from build123d import *

# Parameters (mm, degrees)
BASPROSKE_W         = 6
BASPROSKE_H         = 20.25
TOOTHCUT_DEPTH      = 30.259613805
TEETHCUTS_COUNT     = 25
TEETHCUTS_ANGLE     = 345.6
BORSKE_R            = 0.4
BORE_DEPTH          = 50.0000508
SKETCH1_R           = 0.4
BOSS_EXTRUDE1_DEPTH = 6


with BuildPart() as part:
    # BasProSke → Base-Revolve (revolve)
    with BuildSketch(Plane(origin=(0, 0, 0), x_dir=(1, 0, 0), z_dir=(0, 1, 0)), mode=Mode.PRIVATE) as base_revolve_sk:
        with Locations((3, 10.125)):
            Rectangle(BASPROSKE_W, BASPROSKE_H)
    revolve(base_revolve_sk.sketch.rotate(Axis((-10, 0, 0), (1, 0, 0)), 180), axis=Axis((-10, 0, 0), (1, 0, 0)))

    # TooCutSke → ToothCut (cut, through all)
    with BuildSketch(Plane(origin=(0, 0, 0), x_dir=(0, 0, -1), z_dir=(1, 0, 0))):
        with BuildLine():
            ThreePointArc((0.713909619, 16.858891098), (0, 16.874), (-0.713909619, 16.858891098))
            ThreePointArc((-0.713909619, 16.858891098), (-1.221902209, 18.597177626), (-2.131751691, 20.163022588))
            ThreePointArc((-2.131751691, 20.163022588), (0, 20.2754), (2.131751691, 20.163022588))
            ThreePointArc((2.131751691, 20.163022588), (1.221902209, 18.597177626), (0.713909619, 16.858891098))
        make_face()
    toothcut = extrude(amount=TOOTHCUT_DEPTH, mode=Mode.SUBTRACT)

    # TeethCuts: ToothCut ×25 about axis
    teethcuts_axis = Axis((-10, 0, 0), (1, 0, 0))
    for i in range(1, TEETHCUTS_COUNT):
        add(toothcut.rotate(teethcuts_axis, i * TEETHCUTS_ANGLE / (TEETHCUTS_COUNT - 1)), mode=Mode.SUBTRACT)

    # BorSke → Bore (cut, symmetric)
    with BuildSketch(Plane(origin=(0, 0, 0), x_dir=(0, 0, -1), z_dir=(1, 0, 0))):
        with Locations(Location((0, 0, 0), (0, 0, 180))):
            Circle(BORSKE_R)
    extrude(amount=BORE_DEPTH, both=True, mode=Mode.SUBTRACT)

    # Sketch1 → Boss-Extrude1 (add)
    with BuildSketch(Plane(origin=(6, 0, 0), x_dir=(0, 0, -1), z_dir=(1, 0, 0))):
        with BuildLine():
            ThreePointArc((7.033321313, 19.122578704), (5.755923301, 17.845039552), (4.814939591, 16.302832813))
            ThreePointArc((4.814939591, 16.302832813), (4.227479392, 16.464945156), (3.634585878, 16.605896136))
            ThreePointArc((3.634585878, 16.605896136), (3.55295933, 18.410664563), (3.049026099, 20.145571842))
            ThreePointArc((3.049026099, 20.145571842), (2.553664634, 20.214337039), (2.056764651, 20.270923614))
            ThreePointArc((2.056764651, 20.270923614), (1.137209513, 18.715844736), (0.609319757, 16.988076125))
            ThreePointArc((0.609319757, 16.988076125), (0, 16.999), (-0.609319757, 16.988076125))
            ThreePointArc((-0.609319757, 16.988076125), (-1.137209513, 18.715844736), (-2.056764651, 20.270923614))
            ThreePointArc((-2.056764651, 20.270923614), (-2.553664634, 20.214337039), (-3.049026099, 20.145571842))
            ThreePointArc((-3.049026099, 20.145571842), (-3.55295933, 18.410664563), (-3.634585878, 16.605896136))
            ThreePointArc((-3.634585878, 16.605896136), (-4.227479392, 16.464945156), (-4.814939591, 16.302832813))
            ThreePointArc((-4.814939591, 16.302832813), (-5.755923301, 17.845039552), (-7.033321313, 19.122578704))
            ThreePointArc((-7.033321313, 19.122578704), (-7.500537761, 18.9441959), (-7.963235326, 18.754399701))
            ThreePointArc((-7.963235326, 18.754399701), (-8.019882673, 16.948674626), (-7.650117116, 15.180306621))
            ThreePointArc((-7.650117116, 15.180306621), (-8.189330706, 14.896337254), (-8.718019063, 14.593222558))
            ThreePointArc((-8.718019063, 14.593222558), (-10.012971259, 15.852964904), (-11.567948531, 16.772691847))
            ThreePointArc((-11.567948531, 16.772691847), (-11.976124515, 16.48372126), (-12.37708519, 16.184819653))
            ThreePointArc((-12.37708519, 16.184819653), (-11.982887291, 14.421737129), (-11.18496336, 12.800882612))
            ThreePointArc((-11.18496336, 12.800882612), (-11.636616254, 12.391737698), (-12.073313334, 11.966666459))
            ThreePointArc((-12.073313334, 11.966666459), (-13.640867407, 12.864790167), (-15.375718999, 13.368915074))
            ThreePointArc((-15.375718999, 13.368915074), (-15.699207322, 12.987513791), (-16.013237272, 12.598287862))
            ThreePointArc((-16.013237272, 12.598287862), (-15.192963031, 10.988628849), (-14.01701722, 9.61713207))
            ThreePointArc((-14.01701722, 9.61713207), (-14.352730406, 9.108519688), (-14.669996926, 8.588200696))
            ThreePointArc((-14.669996926, 8.588200696), (-16.411657689, 9.068273351), (-18.217376494, 9.125120201))
            ThreePointArc((-18.217376494, 9.125120201), (-18.435851194, 8.675253066), (-18.643218764, 8.220159312))
            ThreePointArc((-18.643218764, 8.220159312), (-17.448409029, 6.865064605), (-15.968330338, 5.82910175))
            ThreePointArc((-15.968330338, 5.82910175), (-16.167009721, 5.252979887), (-16.344910658, 4.670106699))
            ThreePointArc((-16.344910658, 4.670106699), (-18.15124316, 4.70196357), (-19.914369225, 4.307960465))
            ThreePointArc((-19.914369225, 4.307960465), (-20.014102734, 3.817894285), (-20.101778256, 3.32552792))
            ThreePointArc((-20.101778256, 3.32552792), (-18.607507316, 2.310143104), (-16.916294533, 1.674807529))
            ThreePointArc((-16.916294533, 1.674807529), (-16.965456357, 1.067376041), (-16.992813542, 0.458572722))
            ThreePointArc((-16.992813542, 0.458572722), (-18.750319268, 0.040212124), (-20.360068898, -0.77988427))
            ThreePointArc((-20.360068898, -0.77988427), (-20.334794592, -1.279356835), (-20.297269091, -1.778058621))
            ThreePointArc((-20.297269091, -1.778058621), (-18.597427484, -2.389933184), (-16.801345729, -2.584721008))
            ThreePointArc((-16.801345729, -2.584721008), (-16.697900975, -3.185294967), (-16.572995455, -3.781775066))
            ThreePointArc((-16.572995455, -3.781775066), (-18.171243857, -4.624065996), (-19.526470563, -5.818726009))
            ThreePointArc((-19.526470563, -5.818726009), (-19.37777652, -6.29622126), (-19.21740786, -6.769923199))
            ThreePointArc((-19.21740786, -6.769923199), (-17.418802888, -6.939841181), (-15.630706582, -6.681842018))
            ThreePointArc((-15.630706582, -6.681842018), (-15.381155065, -7.237822177), (-15.111835113, -7.784500017))
            ThreePointArc((-15.111835113, -7.784500017), (-16.450402366, -8.997797045), (-17.465952269, -10.491955792))
            ThreePointArc((-17.465952269, -10.491955792), (-17.203181482, -10.917470948), (-16.930046218, -11.336408605))
            ThreePointArc((-16.930046218, -11.336408605), (-15.145690844, -11.053693433), (-13.477932654, -10.35911832))
            ThreePointArc((-13.477932654, -10.35911832), (-13.097954614, -10.835570402), (-12.701142593, -11.298096204))
            ThreePointArc((-12.701142593, -11.298096204), (-13.695921594, -12.806163413), (-14.307983958, -14.505937407))
            ThreePointArc((-14.307983958, -14.505937407), (-13.947647283, -14.852735784), (-13.578907507, -15.190585766))
            ThreePointArc((-13.578907507, -15.190585766), (-11.920919342, -14.473001475), (-10.47829065, -13.38549312))
            ThreePointArc((-10.47829065, -13.38549312), (-9.991761504, -13.752479887), (-9.492390573, -14.101791454))
            ThreePointArc((-9.492390573, -14.101791454), (-10.080875698, -15.809871436), (-10.250992395, -17.608457625))
            ThreePointArc((-10.250992395, -17.608457625), (-9.81573111, -17.854748606), (-9.374556097, -18.090282557))
            ThreePointArc((-9.374556097, -18.090282557), (-7.947112637, -16.982917606), (-6.820259107, -15.570808159))
            ThreePointArc((-6.820259107, -15.570808159), (-6.257749271, -15.805270484), (-5.687196742, -16.019419285))
            ThreePointArc((-5.687196742, -16.019419285), (-5.832411307, -17.820187093), (-5.549893279, -19.604573691))
            ThreePointArc((-5.549893279, -19.604573691), (-5.067056451, -19.734881908), (-4.581166851, -19.853300363))
            ThreePointArc((-4.581166851, -19.853300363), (-3.473959616, -18.425734565), (-2.733685602, -16.777752055))
            ThreePointArc((-2.733685602, -16.777752055), (-2.130539637, -16.864957808), (-1.524655424, -16.930488086))
            ThreePointArc((-1.524655424, -16.930488086), (-1.217475063, -18.710794856), (-0.500073957, -20.368862291))
            ThreePointArc((-0.500073957, -20.368862291), (0, -20.375), (0.500073957, -20.368862291))
            ThreePointArc((0.500073957, -20.368862291), (1.217475063, -18.710794856), (1.524655424, -16.930488086))
            ThreePointArc((1.524655424, -16.930488086), (2.130539637, -16.864957808), (2.733685602, -16.777752055))
            ThreePointArc((2.733685602, -16.777752055), (3.473959616, -18.425734565), (4.581166851, -19.853300363))
            ThreePointArc((4.581166851, -19.853300363), (5.067056451, -19.734881908), (5.549893279, -19.604573691))
            ThreePointArc((5.549893279, -19.604573691), (5.832411307, -17.820187093), (5.687196742, -16.019419285))
            ThreePointArc((5.687196742, -16.019419285), (6.257749271, -15.805270484), (6.820259107, -15.570808159))
            ThreePointArc((6.820259107, -15.570808159), (7.947112637, -16.982917606), (9.374556097, -18.090282557))
            ThreePointArc((9.374556097, -18.090282557), (9.81573111, -17.854748606), (10.250992395, -17.608457625))
            ThreePointArc((10.250992395, -17.608457625), (10.080875698, -15.809871436), (9.492390573, -14.101791454))
            ThreePointArc((9.492390573, -14.101791454), (9.991761504, -13.752479887), (10.47829065, -13.38549312))
            ThreePointArc((10.47829065, -13.38549312), (11.920919342, -14.473001475), (13.578907507, -15.190585766))
            ThreePointArc((13.578907507, -15.190585766), (13.947647283, -14.852735784), (14.307983958, -14.505937407))
            ThreePointArc((14.307983958, -14.505937407), (13.695921594, -12.806163413), (12.701142593, -11.298096204))
            ThreePointArc((12.701142593, -11.298096204), (13.097954614, -10.835570402), (13.477932654, -10.35911832))
            ThreePointArc((13.477932654, -10.35911832), (15.145690844, -11.053693433), (16.930046218, -11.336408605))
            ThreePointArc((16.930046218, -11.336408605), (17.203181482, -10.917470948), (17.465952269, -10.491955792))
            ThreePointArc((17.465952269, -10.491955792), (16.450402366, -8.997797045), (15.111835113, -7.784500017))
            ThreePointArc((15.111835113, -7.784500017), (15.381155065, -7.237822177), (15.630706582, -6.681842018))
            ThreePointArc((15.630706582, -6.681842018), (17.418802888, -6.939841181), (19.21740786, -6.769923199))
            ThreePointArc((19.21740786, -6.769923199), (19.37777652, -6.29622126), (19.526470563, -5.818726009))
            ThreePointArc((19.526470563, -5.818726009), (18.171243857, -4.624065996), (16.572995455, -3.781775066))
            ThreePointArc((16.572995455, -3.781775066), (16.697900975, -3.185294967), (16.801345729, -2.584721008))
            ThreePointArc((16.801345729, -2.584721008), (18.597427484, -2.389933184), (20.297269091, -1.778058621))
            ThreePointArc((20.297269091, -1.778058621), (20.334794592, -1.279356835), (20.360068898, -0.77988427))
            ThreePointArc((20.360068898, -0.77988427), (18.750319268, 0.040212124), (16.992813542, 0.458572722))
            ThreePointArc((16.992813542, 0.458572722), (16.965456357, 1.067376041), (16.916294533, 1.674807529))
            ThreePointArc((16.916294533, 1.674807529), (18.607507316, 2.310143104), (20.101778256, 3.32552792))
            ThreePointArc((20.101778256, 3.32552792), (20.014102734, 3.817894285), (19.914369225, 4.307960465))
            ThreePointArc((19.914369225, 4.307960465), (18.15124316, 4.70196357), (16.344910658, 4.670106699))
            ThreePointArc((16.344910658, 4.670106699), (16.167009721, 5.252979887), (15.968330338, 5.82910175))
            ThreePointArc((15.968330338, 5.82910175), (17.448409029, 6.865064605), (18.643218764, 8.220159312))
            ThreePointArc((18.643218764, 8.220159312), (18.435851194, 8.675253066), (18.217376494, 9.125120201))
            ThreePointArc((18.217376494, 9.125120201), (16.411657689, 9.068273351), (14.669996926, 8.588200696))
            ThreePointArc((14.669996926, 8.588200696), (14.352730406, 9.108519688), (14.01701722, 9.61713207))
            ThreePointArc((14.01701722, 9.61713207), (15.192963031, 10.988628849), (16.013237272, 12.598287862))
            ThreePointArc((16.013237272, 12.598287862), (15.699207322, 12.987513791), (15.375718999, 13.368915074))
            ThreePointArc((15.375718999, 13.368915074), (13.640867407, 12.864790167), (12.073313334, 11.966666459))
            ThreePointArc((12.073313334, 11.966666459), (11.636616254, 12.391737698), (11.18496336, 12.800882612))
            ThreePointArc((11.18496336, 12.800882612), (11.982887291, 14.421737129), (12.37708519, 16.184819653))
            ThreePointArc((12.37708519, 16.184819653), (11.976124515, 16.48372126), (11.567948531, 16.772691847))
            ThreePointArc((11.567948531, 16.772691847), (10.012971259, 15.852964904), (8.718019063, 14.593222558))
            ThreePointArc((8.718019063, 14.593222558), (8.189330706, 14.896337254), (7.650117116, 15.180306621))
            ThreePointArc((7.650117116, 15.180306621), (8.019882673, 16.948674626), (7.963235326, 18.754399701))
            ThreePointArc((7.963235326, 18.754399701), (7.500537761, 18.9441959), (7.033321313, 19.122578704))
        make_face()
        with Locations(Location((0, 0, 0), (0, 0, 180))):
            Circle(SKETCH1_R, mode=Mode.SUBTRACT)
    extrude(amount=-BOSS_EXTRUDE1_DEPTH)


solid = part.part
CAD build for the part. Positions are in the model's coordinates, mm. A direction names the side the tool comes from. Give positions to 0.01 mm unless a question says otherwise; leave off trailing zeros. Loops run counter-clockwise (first coordinate to the right, second up) from the corner with the lowest first, then second, coordinate; pieces in that order, holes last. Notation, with made-up numbers: M 28.5,27 L 60.5,27 A6 cw 60.5,31 Z; hole C 75,82 d7. An arc over 180 degrees is marked long. Write each question's results on one line, items separated by ' | '.
Q1. Mould opens along Z. For faces 1 (the face through (6, -4, 0)), 2 (the face through (3.042, 3.811, -20.015)), 3 (the face through (3.04, 12.4, 11.63)) say: pulls with the +Z half, pulls with the -Z half, needs draft (parallel to the pull), parting line crosses it, or undercut.
Geometry check:
face 1: needs draft | face 2: pulls with the -Z half | face 3: undercut
Q2. Band-saw the part on A-A on y = 11.5. Write the cut outline in (x, z).
Geometry check:
outline: M 0,-15.51 L 6,-15.51 L 6,15.51 L 0,15.51 Z
Q3. Band-saw the part on B-B on y = 6.5. Write the cut outline in (x, z).
Geometry check:
outline: M 0,-17.01 L 6,-17.01 L 6,17.01 L 0,17.01 Z
Q4. Probe probe 1 along Y at (x, z) = (2.6, 0) (3 decimals); probe 2 along Y at (x, z) = (3.6, 17.5); probe 3 along Z at (x, y) = (2.2, 16). List the from-to ranges inside material, lowest first.
Geometry check:
probe 1: y = -20.375 to -0.4, 0.4 to 16.999 | probe 2: y = -6.94 to -4.21, -2.56 to 0.38, 1.84 to 4.74, 6.91 to 9.15 | probe 3: z = -12.36 to -10.21, -7.88 to 7.88, 10.21 to 12.36
Q5. Which spindle directions (+Z, -Z, +X, -X, +Y, -Y) get a long thin tool onto all of the face, cutting with end or side? Do faces 4 (the face through (3, 11, -15.2)), 5 (the face through (3.042, 14.446, 11.991)), 6 (the face through (3.042, 17.825, 5.74)). Say none if no direction does.
Geometry check:
face 4: -Z, +X, -X | face 5: +X, -X | face 6: +X, -X, +Y
Q6. Flat gauge pins, fed straight in: P1, Ø1, axis at x = 2, z = -7.5, coming from the -Y side; P2, Ø3, axis at y = 13.5, z = -5, coming from the -X side; P3, Ø1.5, axis at x = 5.5, z = 11.5, coming from the +Y side. Where does each tip first touch, or does it go through?
Geometry check:
P1: stops at y = -17.03 | P2: stops at x = 0 | P3: stops at y = 16.77
